Autodesk Fusion 360 part; units mm, degrees
sketch "Sketch2" plane through (0, 0, 0) normal (0, 1, 0) x (1, 0, 0)
  line L0 (-80, -90) -> (100, -90)
  line L1 (100, -90) -> (100, 90)
  line L2 (100, 90) -> (-80, 90)
  line L3 (-80, 90) -> (-80, -90)
  dimension "d3" = 180
  dimension "d4" = 180
extrude "Extrude1" add sketch "Sketch2" along normal blind 100
sketch "Sketch3" plane through (0, 100, 0) normal (0, 1, 0) x (-1, 0, 0)
  line L0 (80, -90) -> (80, 90)
  line L1 (80, 90) -> (-100, 90)
  line L2 (-100, 90) -> (-100, -90)
  line L3 (-100, -90) -> (80, -90)
  line L4 (75, -85) -> (-95, -85)
  line L5 (-95, -85) -> (-95, 85)
  line L6 (-95, 85) -> (75, 85)
  line L7 (75, 85) -> (75, -85)
extrude "Extrude2" cut sketch "Sketch3" against normal blind 5 contours L4 L5 L6 L7
sketch "Sketch4" plane through (0, 95, 0) normal (0, 1, 0) x (-1, 0, 0)
  line L0 (75, 85) -> (-95, 85)
  line L1 (-95, 85) -> (-95, -85)
  line L2 (-95, -85) -> (75, -85)
  line L3 (75, -85) -> (75, 85)
  line L4 (70, 80) -> (-90, 80)
  line L5 (-90, 80) -> (-90, -80)
  line L6 (-90, -80) -> (70, -80)
  line L7 (70, -80) -> (70, 80)
extrude "Extrude3" cut sketch "Sketch4" against normal blind 175 contours L4 L5 L6 L7
sketch "Sketch5" plane through (0, 0, 0) normal (0, -1, 0) x (1, 0, 0)
  line L0 (-70, 80) -> (90, 80)
  line L1 (90, 80) -> (90, -80)
  line L2 (90, -80) -> (-70, -80)
  line L3 (-70, -80) -> (-70, 80)
  line L4 (-80, 90) -> (-80, -90)
  line L5 (-80, -90) -> (100, -90)
  line L6 (100, -90) -> (100, 90)
  line L7 (100, 90) -> (-80, 90)
  line L8 (95, -85) -> (-75, -85)
  line L9 (-75, -85) -> (-75, 85)
  line L10 (-75, 85) -> (95, 85)
  line L11 (95, 85) -> (95, -85)
  point P0 (95, -85)
  point P1 (-75, 85)
extrude "Extrude4" cut sketch "Sketch5" against normal blind 5 contours L8 L9 L10 L11
sketch "Sketch6" plane through (0, 0, 0) normal (0, -1, 0) x (1, 0, 0)
  line L0 (-75, -85) -> (-75, 85)
  line L1 (-75, 85) -> (95, 85)
  line L2 (95, 85) -> (95, -85)
  line L3 (95, -85) -> (-75, -85)
  line L4 (-80, 90) -> (-80, -90)
  line L5 (-80, -90) -> (100, -90)
  line L6 (100, -90) -> (100, 90)
  line L7 (100, 90) -> (-80, 90)
  line L8 (95, -85) -> (85, -85)
  line L9 (85, -85) -> (85, -75)
  line L10 (85, -75) -> (95, -75)
  line L11 (95, -75) -> (95, -85)
  dimension "d13" = 10
extrude "Extrude5" cut sketch "Sketch6" against normal blind 10 contours L2 L3 L8 L9 L10 L11
sketch "Sketch7" plane through (0, 5, 0) normal (0, -1, 0) x (1, 0, 0)
  line L0 (90, -75) -> (95, -75)
  line L1 (95, -75) -> (95, 85)
  line L2 (95, 85) -> (-75, 85)
  line L3 (-75, 85) -> (-75, -85)
  line L4 (-75, -85) -> (85, -85)
  line L5 (85, -85) -> (85, -80)
  line L6 (85, -80) -> (-70, -80)
  line L7 (-70, -80) -> (-70, 80)
  line L8 (-70, 80) -> (90, 80)
  line L9 (90, 80) -> (90, -75)
  line L10 (95, 85) -> (85, 85)
  line L11 (85, 85) -> (85, 75)
  line L12 (85, 75) -> (95, 75)
  line L13 (95, 75) -> (95, 85)
extrude "Extrude6" cut sketch "Sketch7" against normal blind 10 contours L1 L2 L8 L9 L10 L11 L12 L13
sketch "Sketch8" plane through (0, 5, 0) normal (0, -1, 0) x (1, 0, 0)
  line L0 (85, 80) -> (85, 85)
  line L1 (85, 85) -> (-75, 85)
  line L2 (-75, 85) -> (-75, -85)
  line L3 (-75, -85) -> (85, -85)
  line L4 (85, -85) -> (85, -80)
  line L5 (85, -80) -> (-70, -80)
  line L6 (-70, -80) -> (-70, 80)
  line L7 (-70, 80) -> (85, 80)
  line L8 (-75, -85) -> (-65, -85)
  line L9 (-65, -85) -> (-65, -75)
  line L10 (-65, -75) -> (-75, -75)
  line L11 (-75, -75) -> (-75, -85)
extrude "Extrude7" cut sketch "Sketch8" against normal blind 10 contours L2 L3 L5 L6 L8 L9 L10 L11
sketch "Sketch9" plane through (0, 5, 0) normal (0, -1, 0) x (1, 0, 0)
  line L0 (-75, -75) -> (-70, -75)
  line L1 (-70, -75) -> (-70, 80)
  line L2 (-70, 80) -> (85, 80)
  line L3 (85, 80) -> (85, 85)
  line L4 (85, 85) -> (-75, 85)
  line L5 (-75, 85) -> (-75, -75)
  line L6 (-75, 85) -> (-65, 85)
  line L7 (-65, 85) -> (-65, 75)
  line L8 (-65, 75) -> (-75, 75)
  line L9 (-75, 75) -> (-75, 85)
extrude "Extrude8" cut sketch "Sketch9" against normal blind 10 contours L1 L2 L4 L5 L6 L7 L8 L9
sketch "Sketch11" plane through (-75, 0, 0) normal (1, 0, 0) x (0, 0, -1)
  line L0 (85, 100) -> (-85, 100)
  line L1 (-85, 100) -> (-85, 95)
  line L2 (-85, 95) -> (85, 95)
  line L3 (85, 95) -> (85, 100)
Design review of the part built by this model. Coordinates are the model's own, in mm. A direction names the side the tool comes from. Give positions to 0.01 mm unless a question says otherwise; leave off trailing zeros. Write each loop counter-clockwise with the first axis right and the second up, starting at its lowest first coordinate (ties: lowest second). Pieces come first, ordered by that corner, then holes. Notation, with made-up numbers: (72, -29) - (87, -29) arc R32 cw to (87, 7) - close; hole circle Ø11 at (80, 26.5). An arc over 180 degrees is marked (long way). Return JSON: item names as keys, results as strings. Group by question number.
(1) Insertion check: pin 1 (3 mm diameter, centred on x = -70.5, z = -78.5, fed in from -Y). The pin has a flat end and moves straight along its axis. Give the tip position at first contact, or say it passes through.
(2) We need section C-C, the plane x = 28.5. Give the boundary of the cut face in (y, z).
(3) We need section B-B, the plane y = 23. Give the boundary of the cut face in (x, z), then the cut area to 3 significant figures.
(4) To check wall thickness, follow probe 1 along X at (y, z) = (41, -0.5); probe 2 along Z at (x, y) = (-8, 87.5); probe 3 along Y at (x, z) = (-70.5, 49). State the ranges of each line that lie inside material, in increasing order.
(5) Mouldability with a two-part tool opening along X and no side actions: class faces 1 (the flat face through (100, 49, 1)), 2 (the flat face through (92, 7, -75)), 3 (the flat face through (9, 49, 90)) as +X half, -X half, draft (parallel to the pull), parting line (faces both ways), or undercut.
(6) We need section A-A, the plane z = -77.5. Give the boundary of the cut face in (x, y), then the cut area to 4 significant figures.
(7) Machinability: for faces 4 (the flat face through (3, 0, 86)), 5 (the flat face through (-10, 4, 85)), 6 (the flat face through (-75, 98, 1)), 7 (the flat face through (-80, 49, -1)), 8 (the flat face through (-70, 51, -1)), which of the approach directions +Z, -Z, +X, -X, +Y, -Y give a long, thin tool a straight path to every point of the face, cutting with its end or side? Answer none if there is none.
Reported:
{
 "1": {"pin 1": "stops at y = 15"},
 "2": {"outline": "(0, -90) - (100, -90) - (100, -85) - (95, -85) - (95, -80) - (5, -80) - (5, -85) - (0, -85) - close; (0, 85) - (5, 85) - (5, 80) - (95, 80) - (95, 85) - (100, 85) - (100, 90) - (0, 90) - close"},
 "3": {"outline": "(-80, -90) - (100, -90) - (100, 90) - (-80, 90) - close; hole (-70, -80) - (90, -80) - (90, 80) - (-70, 80) - close", "area": "6,800 mm2"},
 "4": {"probe 1": "x = -80 to -70, 90 to 100", "probe 2": "z = -90 to -80, 80 to 90", "probe 3": "y = 5 to 95"},
 "5": {"face 1": "+X half", "face 2": "undercut", "face 3": "draft"},
 "6": {"outline": "(-80, 0) - (-75, 0) - (-75, 15) - (-70, 15) - (-70, 95) - (-75, 95) - (-75, 100) - (-80, 100) - close; (90, 10) - (95, 10) - (95, 0) - (100, 0) - (100, 100) - (95, 100) - (95, 95) - (90, 95) - close", "area": "1,825 mm2"},
 "7": {"face 4": "+Z, -Z, +X, -X, -Y", "face 5": "-Y", "face 6": "+Y", "face 7": "+Z, -Z, -X, +Y, -Y", "face 8": "+Y, -Y"}
}
